```python
from build123d import *

# Parameters (mm, degrees)
SKETCH_1_W      = 460
SKETCH_1_H      = 30
SKETCH_1_R      = 6
EXTRUDE_1_DEPTH = 2.5
FILLET_1_RADIUS = 15
FILLET_1_LENGTH = 5
SKETCH_3_R      = 15
EXTRUDE_2_DEPTH = 25
SKETCH_4_R      = 6
EXTRUDE_3_DEPTH = 35


with BuildPart() as part:
    # 草图1 → 凸台-拉伸1 (new, symmetric)
    with BuildSketch(Plane.XY):
        Rectangle(SKETCH_1_W, SKETCH_1_H)
        with Locations((-220, 0)):
            Circle(SKETCH_1_R, mode=Mode.SUBTRACT)
        with Locations((220, 0)):
            Circle(SKETCH_1_R, mode=Mode.SUBTRACT)
    extrude(amount=EXTRUDE_1_DEPTH, both=True)

    # 圆角1: full round fillet: the end face becomes a half cylinder, R = half its width
    fillet_1_face = Plane((-230, 0, 0), x_dir=(0, 0, 1), z_dir=(-1, 0, 0))  # on the end face: x along it, z out of the body
    fillet_1_slab = fillet_1_face.offset(-FILLET_1_RADIUS / 2) * Box(FILLET_1_LENGTH, 2 * FILLET_1_RADIUS, FILLET_1_RADIUS, mode=Mode.PRIVATE)  # the body's end, R deep
    fillet_1_round = Plane((-215, 0, 0), x_dir=(-1, 0, 0), z_dir=(0, 0, 1)) * Cylinder(FILLET_1_RADIUS, FILLET_1_LENGTH, mode=Mode.PRIVATE)  # its axis R under the face
    add(fillet_1_slab - fillet_1_round, mode=Mode.SUBTRACT)

    # 草图3 → 凸台-拉伸2 (add, symmetric)
    with BuildSketch(Plane.XY):
        with Locations((-215, 0)):
            Circle(SKETCH_3_R)
    extrude(amount=EXTRUDE_2_DEPTH, both=True)

    # 草图4 → 凸台-拉伸3 (add, symmetric)
    with BuildSketch(Plane.XY):
        with Locations((-215, 0)):
            Circle(SKETCH_4_R)
    extrude(amount=EXTRUDE_3_DEPTH, both=True)


solid = part.part
```
The listing builds one solid part. Answer for the finished solid, in the listing's coordinates (mm). A direction names the side the tool comes from. Round coordinates to 2 decimals unless told otherwise and drop trailing zeros. Loops run counter-clockwise (first coordinate to the right, second up) from the corner with the lowest first, then second, coordinate; pieces in that order, holes last. Notation, with made-up numbers: (80, 21.25) - (101, 21.25) arc R28 ccw to (101, 49.25) - close; hole circle Ø11 at (58, 14.5). An arc over 180 degrees is marked (long way). Use one line per item in the form item = value. Start each with the question number.
1. The part is cut by section C-C on z = -9. Determine the outline of the cut face in (x, y).
2. For a pull along Y with two mould halves and no side action, classify faces 4 (the face through (4, 0, 2.5)), 5 (the face through (225.723, 1.802, -0.035)), 6 (the face through (-219.76, -3.65, 30.07)) as pulls with the +Y half, pulls with the -Y half, needs draft (parallel to the pull), parting line crosses it, or undercut.
3. Given pin 1 Ø1.5 at (y, z) = (-5.5, -6) entering from +X; pin 2 Ø14 at (x, y) = (220, 0) entering from +Z; pin 3 Ø12 at (x, z) = (61, -13.5) entering from +Y; pin 4 Ø15 at (x, y) = (117, 1.5) entering from -Z, each flat-ended and moving along its own axis, determine where each tip first touches the part or whether it passes through.
4. Consider line 1 (Y direction, x = 220, z = 0.65); line 2 (Z direction, x = 157.5, y = 13.25); line 3 (X direction, y = 13.75, z = -19.5). Determine where each line is inside the solid, lowest interval first. Write a range as [from, to].
5. The part is cut by section D-D on x = -170. Determine the outline of the cut face in (y, z).
6. A tool of negligible diameter and unlimited length cuts with its end or side. For faces 1 (the face through (-215, 0, 35)), 2 (the face through (-208.5, 0.2, 25)), 3 (the face through (-219.76, -3.65, -29.93)), from which of +Z, -Z, +X, -X, +Y, -Y can it reach the whole face along a straight path? Write none if from no direction.
7. The part is cut by section A-A on x = 220. Determine the outline of the cut face in (y, z).
8. The part is cut by section B-B on y = 0. Determine the outline of the cut face in (x, z), then the cut area to 3 significant figures.
Geometry check:
q1.outline = circle Ø30 at (-215, 0)
q2.face_4 = needs draft
q2.face_5 = undercut
q2.face_6 = parting line crosses it
q3.pin_1 = -200.77
q3.pin_2 = 2.5
q3.pin_3 = through
q3.pin_4 = -2.5
q4.line_1 = [-15, -6], [6, 15]
q4.line_2 = [-2.5, 2.5]
q4.line_3 = [-220.99, -209.01]
q5.outline = (-15, -2.5) - (15, -2.5) - (15, 2.5) - (-15, 2.5) - close
q6.face_1 = +Z, +X, -X, +Y, -Y
q6.face_2 = +Z
q6.face_3 = -Z
q7.outline = (-15, -2.5) - (-6, -2.5) - (-6, 2.5) - (-15, 2.5) - close; (6, -2.5) - (15, -2.5) - (15, 2.5) - (6, 2.5) - close
q8.outline = (-230, -25) - (-221, -25) - (-221, -35) - (-209, -35) - (-209, -25) - (-200, -25) - (-200, -2.5) - (214, -2.5) - (214, 2.5) - (-200, 2.5) - (-200, 25) - (-209, 25) - (-209, 35) - (-221, 35) - (-221, 25) - (-230, 25) - close; (226, -2.5) - (230, -2.5) - (230, 2.5) - (226, 2.5) - close
q8.area = 3,830 mm^2
